from build123d import *

# Parameters (mm, degrees)
F0_W     = 25.4
F0_H     = 25.4
F1_DEPTH = 12.7
F3_DEPTH = 25.4
F5_R     = 1.5875


# Not quite as in the source:
# - a feature names something its author has since deleted; it is built from what else it names


with BuildPart() as f1:
    # F0 (on Front) → F1 (new body)
    with BuildSketch(Plane.XZ):
        with Locations((12.7, 12.7)):
            Rectangle(F0_W, F0_H)
    extrude(amount=F1_DEPTH)

    # F2 (on face) → F3 (cut)
    with BuildSketch(Plane.XZ.offset(12.7)):
        Polygon((25.4, 5.08), (25.4, 20.32), (7.62, 20.32), (7.62, 15.24), (15.1830166578, 15.24), (15.1830166578, 10.16), (7.62, 10.16), (7.62, 5.08), align=None)
    extrude(amount=-F3_DEPTH, mode=Mode.SUBTRACT)

    # F5 (on offset) → F6 (revolve)
    with BuildSketch(Plane.XZ.offset(6.35)):
        with Locations((12.7, 25.4)):
            Circle(F5_R)
    revolve(axis=Axis((14.955827035, -6.35, 28.575), (1, 0, 0)))


solid = f1.part
Design review of the part built by this model. Coordinates are the model's own, in mm. A direction names the side the tool comes from. Give positions to 0.01 mm unless a question says otherwise; leave off trailing zeros. Loops run counter-clockwise (first coordinate to the right, second up) from the corner with the lowest first, then second, coordinate; pieces in that order, holes last. Notation, with made-up numbers: (88, 62) - (145, 62) arc R8 ccw to (145, 72) - close; hole circle Ø7 at (18, -38.5). An arc over 180 degrees is marked (long way). Write item = value, one per line.
1) Clearance check with flat-ended pins moving along their axes: pin 1 Ø1 at (x, z) = (5.5, 26) entering from -Y; pin 2 Ø5 at (y, z) = (-8.5, 28.5) entering from -X; pin 3 Ø4 at (x, y) = (18.5, -4) entering from +Z; pin 4 Ø1.5 at (y, z) = (-6.5, 13.5) entering from +X. State where each tip first meets the part, or that it passes through.
Result sheet:
pin_1 = through
pin_2 = 11.11
pin_3 = 25.4
pin_4 = 15.18
2) To check wall thickness, follow line 1 (Z direction, x = 11.75, y = -11.5); line 2 (Z direction, x = 23, y = -9); line 3 (Z direction, x = 13, y = -4.5). State the ranges of each line that lie inside material, in increasing order.
Result sheet:
line_1 = 0 to 5.08, 10.16 to 15.24, 20.32 to 25.4
line_2 = 0 to 5.08, 20.32 to 25.4
line_3 = 0 to 5.08, 10.16 to 15.24, 20.32 to 32.93
3) Draft analysis for pull direction Z (two halves, no side actions). For faces 3 (the face through (13, -6, 0)), 4 (the face through (7.62, -6, 8)), 5 (the face through (10, -12.7, 13)), state which applies: +Z half, -Z half, draft (parallel to the pull), parting line (faces both ways), or undercut.
Result sheet:
face_3 = -Z half
face_4 = undercut
face_5 = draft
4) Take a section at C-C on z = 14. State the section outline as (x, y) points.
Result sheet:
outline = (0, -12.7) - (15.18, -12.7) - (15.18, 0) - (0, 0) - close
5) Take a section at A-A on x = 9.75. State the section outline as (y, z) points, and give its area (3 significant figures).
Result sheet:
outline = (-12.7, 0) - (0, 0) - (0, 5.08) - (-12.7, 5.08) - close; (-12.7, 10.16) - (0, 10.16) - (0, 15.24) - (-12.7, 15.24) - close; (-12.7, 20.32) - (0, 20.32) - (0, 25.4) - (-12.7, 25.4) - close
area = 194 mm2
6) Take a section at B-B on x = 16.75. State the section outline as (y, z) points.
Result sheet:
outline = (-12.7, 0) - (0, 0) - (0, 5.08) - (-12.7, 5.08) - close; (-12.7, 20.32) - (0, 20.32) - (0, 25.4) - (-12.7, 25.4) - close
7) Take a section at D-D on x = 2.75. State the section outline as (y, z) points.
Result sheet:
outline = (-12.7, 0) - (0, 0) - (0, 25.4) - (-12.7, 25.4) - close
8) Tool access review of faces 1 (the face through (25.4, -6, 23)), 2 (the face through (7.62, -6, 18)): name each direction out of +Z, -Z, +X, -X, +Y, -Y from which nothing blocks a thin tool from reaching the whole face with its end or side.
Result sheet:
face_1 = +Z, -Z, +X, +Y, -Y
face_2 = +X, +Y, -Y
